Can you work these out from the model? Positions are in its coordinate system, mm. Face numbers are marked on the shaded views. A direction names the side the tool comes from. Round coordinates to 2 decimals unless told otherwise and drop trailing zeros. Order: outer loops, then holes, each group sorted by start corner. A loop starts at its lowest first (then second) coordinate and runs counter-clockwise, first axis right, second up.
Q1. If we section it at C-C (z = 16.5): Please give me the cut outline in (x, y).
Q2. If we section it at B-B (y = -75.5): Please give me the cut outline in (x, z).
Q3. We'd pull the mould along Y, two halves only. Please class the marked faces 1, 2 and 3: pulls with the +Y half, pulls with the -Y half, needs draft (parallel to the pull), parting line crosses it, or undercut.
Q4. If I drill on line 1 (Y direction, x = 0, z = 9); line 2 (Y direction, x = -7, z = 17) (3 decimals); line 3 (X direction, y = -111, z = 1.5), over which ranges is the centre line in solid material (lowest first)?
Q5. For the marked faces 4 and 5, which set-ups out of +Z, -Z, +X, -X, +Y, -Y let a thin tool reach every point of the face, with its end or its side?
Q6. Will these pins go through, and if not, where does the flat tip stop? P1, Ø12, axis at y = -10, z = 8, coming from the -X side; P2, Ø16, axis at x = 0, y = 0, coming from the -Z side; P3, Ø12, axis at x = -9, z = 6, coming from the -Y side; P4, Ø10, axis at x = 13, z = 7, coming from the +Y side.
Q7. If we section it at A-A (x = 0): Please give me the cut outline in (y, z), plus the area to 3 significant figures.
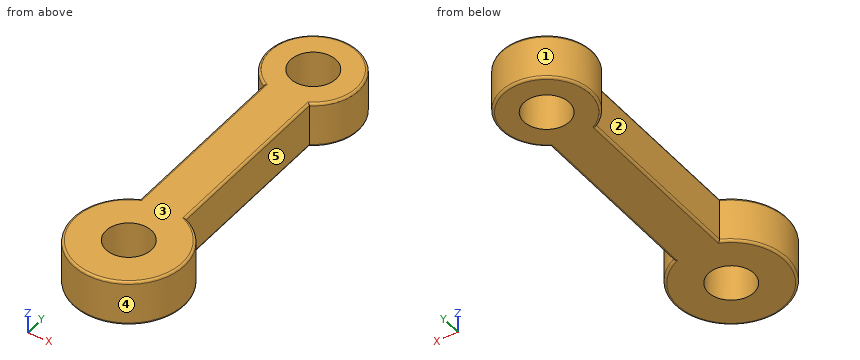
from build123d import *

# Parameters (mm, degrees)
ESQUISSE1_R        = 10
BOSS_EXTRU_1_DEPTH = 20
CONG_2_R           = 1


with BuildPart() as part:
    # Esquisse1 → Boss.-Extru.1 (new body)
    with BuildSketch(Plane.XY):
        with BuildLine():
            Line((-10, -17.320508076), (-10, -97.320508076))
            ThreePointArc((-10, -97.320508076), (0, -144.099247501), (10, -97.320508076))
            Line((10, -97.320508076), (10, -17.320508076))
            ThreePointArc((10, -17.320508076), (0, 20), (-10, -17.320508076))
        make_face()
        Circle(ESQUISSE1_R, mode=Mode.SUBTRACT)
        with Locations((0, -119.641016151)):
            Circle(ESQUISSE1_R, mode=Mode.SUBTRACT)
    extrude(amount=BOSS_EXTRU_1_DEPTH)

    # Congé2
    cong_2_edges = [part.edges().sort_by_distance(p)[0] for p in [
        (0, -144.099247501, 20),
        (10, -57.320508076, 20),
        (0, 20, 20),
        (10, -57.320508076, 0),
        (0, -144.099247501, 0),
        (-10, -57.320508076, 0),
        (0, 20, 0),
        (-10, -57.320508076, 20),
    ]]
    fillet(cong_2_edges, radius=CONG_2_R)


solid = part.part
Solution:
1. outline: (-10, -97.32) arc R24.46 ccw (long way) to (10, -97.32) - (10, -17.32) arc R20 ccw (long way) to (-10, -17.32) - close; hole circle Ø20 at (0, -119.64); hole circle Ø20 at (0, 0)
2. outline: (-10, 1) arc R1 ccw to (-9, 0) - (9, 0) arc R1 ccw to (10, 1) - (10, 19) arc R1 ccw to (9, 20) - (-9, 20) arc R1 ccw to (-10, 19) - close
3. face 1: undercut
3. face 2: undercut
3. face 3: needs draft
4. line 1: y = -144.1 to -129.64, -109.64 to -10, 10 to 20
4. line 2: y = -143.076 to -126.782, -112.5 to -7.141, 7.141 to 18.735
4. line 3: x = -22.88 to -5.03, 5.03 to 22.88
5. face 4: +Z, -Z
5. face 5: +Z, -Z, +X
6. P1: stops at x = -19.6
6. P2: passes through
6. P3: stops at y = -143.91
6. P4: stops at y = 18.33
7. outline: (-144.1, 1) arc R1 ccw to (-143.1, 0) - (-129.64, 0) - (-129.64, 20) - (-143.1, 20) arc R1 ccw to (-144.1, 19) - close; (-109.64, 0) - (-10, 0) - (-10, 20) - (-109.64, 20) - close; (10, 0) - (19, 0) arc R1 ccw to (20, 1) - (20, 19) arc R1 ccw to (19, 20) - (10, 20) - close
7. area: 2,480 mm2
